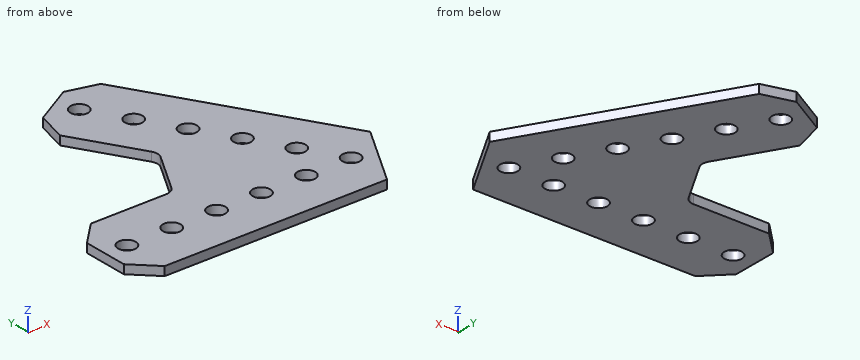
from build123d import *

# Parameters (mm, degrees)
SKETCH1_R           = 2.5
BOSS_EXTRUDE1_DEPTH = 2.5


with BuildPart() as part:
    # Sketch1 → Boss-Extrude1 (new body)
    with BuildSketch(Plane(origin=(0, 0, -1.25), x_dir=(-1, 0, 0), z_dir=(0, 0, -1))):
        with BuildLine():
            Line((0.293293937, -12.7), (63.246, -12.7))
            Line((63.246, -12.7), (69.596, -6.35))
            Line((69.596, -6.35), (69.596, 6.35))
            Line((69.596, 6.35), (63.246, 12.7))
            Line((63.246, 12.7), (41.897783942, 12.7))
            ThreePointArc((41.897783942, 12.7), (40.310283942, 13.125369343), (39.148153285, 14.2875))
            Line((39.148153285, 14.2875), (31.947414599, 26.759545256))
            ThreePointArc((31.947414599, 26.759545256), (31.522045256, 28.347045256), (31.947414599, 29.934545256))
            Line((31.947414599, 29.934545256), (42.621522628, 48.422642688))
            Line((42.621522628, 48.422642688), (40.297261314, 57.096904002))
            Line((40.297261314, 57.096904002), (29.298738686, 63.446904002))
            Line((29.298738686, 63.446904002), (20.624477372, 61.122642688))
            Line((20.624477372, 61.122642688), (-10.85187566, 6.604))
            Line((-10.85187566, 6.604), (0.293293937, -12.7))
        make_face()
        with Locations((12.7, 0)):
            Circle(SKETCH1_R, mode=Mode.SUBTRACT)
        with Locations((25.4, 0)):
            Circle(SKETCH1_R, mode=Mode.SUBTRACT)
        with Locations((38.1, 0)):
            Circle(SKETCH1_R, mode=Mode.SUBTRACT)
        Circle(SKETCH1_R, mode=Mode.SUBTRACT)
        with Locations((63.5, 0)):
            Circle(SKETCH1_R, mode=Mode.SUBTRACT)
        with Locations((50.8, 0)):
            Circle(SKETCH1_R, mode=Mode.SUBTRACT)
        with Locations((31.75, 54.99261314)):
            Circle(SKETCH1_R, mode=Mode.SUBTRACT)
        with Locations((25.4, 43.994090512)):
            Circle(SKETCH1_R, mode=Mode.SUBTRACT)
        with Locations((19.05, 32.995567884)):
            Circle(SKETCH1_R, mode=Mode.SUBTRACT)
        with Locations((12.7, 21.997045256)):
            Circle(SKETCH1_R, mode=Mode.SUBTRACT)
        with Locations((6.35, 10.998522628)):
            Circle(SKETCH1_R, mode=Mode.SUBTRACT)
    extrude(amount=-BOSS_EXTRUDE1_DEPTH)


solid = part.part
Can you work these out from the model? Positions are in its coordinate system, mm. Give positions to 0.01 mm unless a question says otherwise; leave off trailing zeros. Loops run counter-clockwise (first coordinate to the right, second up) from the corner with the lowest first, then second, coordinate; pieces in that order, holes last. Notation, with made-up numbers: M -21,-20 L 24,-20 A21 ccw 24,-8 Z; hole C 43,73 d9. An arc over 180 degrees is marked long. One line per item, written item: value. Start each with the question number.
1) I'm going to push a flat-ended pin straight in: pin 1 (1.5 mm diameter, centred on y = 21, z = 0.5, fed in from -X). Where does the tip first touch, or does it pass through?
2) If we section it at B-B, the plane y = 0: Write out the boundary of the cut face in (x, z).
3) If I drill on line 1 (Y direction, x = -25.4, z = -0.3); line 2 (Y direction, x = -59, z = 0.85); line 3 (Y direction, x = -39.5, z = -0.7), over which ranges is the centre line in solid material (lowest first)? Write a range as [from, to].
4) If we section it at C-C, the plane x = -25: Write out the boundary of the cut face in (y, z), and give its area (3 significant figures).
5) If we section it at A-A, the plane x = -50.8: Write out the boundary of the cut face in (y, z), and give its area (3 significant figures).
6) If we section it at D-D, the plane z = -0.85: Give the number of separate pieces and of enclosed holes in the cut face, and give its area (3 significant figures).
Completed:
1. pin 1: stops at x = -35.71
2. outline: M -69.6,-1.25 L -66,-1.25 L -66,1.25 L -69.6,1.25 Z; M -61,-1.25 L -53.3,-1.25 L -53.3,1.25 L -61,1.25 Z; M -48.3,-1.25 L -40.6,-1.25 L -40.6,1.25 L -48.3,1.25 Z; M -35.6,-1.25 L -27.9,-1.25 L -27.9,1.25 L -35.6,1.25 Z; M -22.9,-1.25 L -15.2,-1.25 L -15.2,1.25 L -22.9,1.25 Z; M -10.2,-1.25 L -2.5,-1.25 L -2.5,1.25 L -10.2,1.25 Z; M 2.5,-1.25 L 7.04,-1.25 L 7.04,1.25 L 2.5,1.25 Z
3. line 1: y = [-12.7, -2.5], [2.5, 41.49], [46.49, 62.4]
3. line 2: y = [-12.7, 12.7]
3. line 3: y = [-12.7, -2.07], [2.07, 13.79], [43.02, 57.56]
4. outline: M -12.7,-1.25 L -2.47,-1.25 L -2.47,1.25 L -12.7,1.25 Z; M 2.47,-1.25 L 41.53,-1.25 L 41.53,1.25 L 2.47,1.25 Z; M 46.46,-1.25 L 62.3,-1.25 L 62.3,1.25 L 46.46,1.25 Z
4. area: 163 mm^2
5. outline: M -12.7,-1.25 L -2.5,-1.25 L -2.5,1.25 L -12.7,1.25 Z; M 2.5,-1.25 L 12.7,-1.25 L 12.7,1.25 L 2.5,1.25 Z
5. area: 51.0 mm^2
6. separate pieces: 1
6. enclosed holes: 11
6. area: 3,170 mm^2
